Geometry: final body of the model. Coordinates: model frame, mm. Face numbers are marked on the shaded views. A direction names the side the tool comes from. Give positions to 0.01 mm unless a question says otherwise; leave off trailing zeros. Order: outer loops, then holes, each group sorted by start corner. A loop starts at its lowest first (then second) coordinate and runs counter-clockwise, first axis right, second up. Notation, with made-up numbers: (-31, 11) - (21, 11) arc R27 cw to (21, 36) - close; hole circle Ø8 at (51.5, 89.25). An arc over 180 degrees is marked (long way). Put each result on its own line as item: value. Start each with the question number.
1. Ray query, line 1 along Y through (x, z) = (0, -20.25); line 2 along X through (y, z) = (15, 20.5); line 3 along Z through (x, y) = (-3.25, 9.5). Return the intervals inside material, ascending. Write a range as from..to.
2. Set-up query: the marked faces 4 and 5. Return all of +Z, -Z, +X, -X, +Y, -Y with unobstructed straight access to the full face (end or side cutting, diameter ignored); none if empty.
3. First-contact query: P1, Ø2.5, axis at x = 0, y = 8.3, coming from the +Z side; P2, Ø3, axis at x = 3.5, z = -11, coming from the +Y side. Flat tips, straight axial feed; report the tip coordinate or a pass-through.
4. Section B-B on y = 17.5. Return the cut outline in (x, z), plus the area to 3 significant figures.
5. Section C-C on y = 15. Return the cut outline in (x, z), plus the area to 3 significant figures.
6. Section A-A on x = 0. Return the cut outline in (y, z), plus the area to 3 significant figures.
7. Mould query, pull axis Z, two halves, no side actions, for the marked faces 1, 2 and 3. Classes: pulls with the +Z half, pulls with the -Z half, needs draft (parallel to the pull), parting line crosses it, or undercut.
8. Section D-D on x = 3.5. Return the cut outline in (y, z).
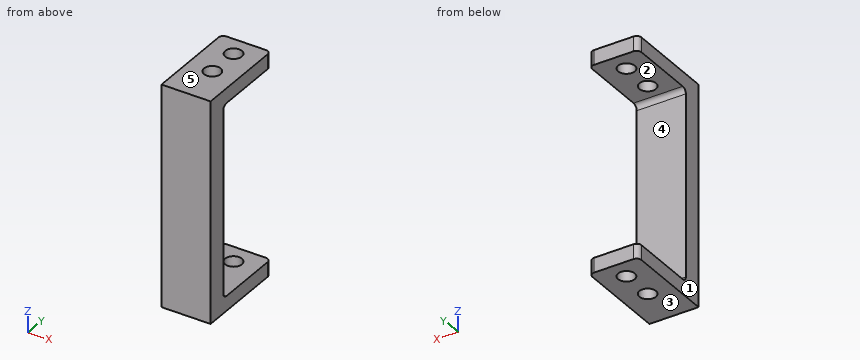
from build123d import *

# Parameters (mm, degrees)
SKETCH2_W                      = 10
SKETCH2_H                      = 45
BOSS_EXTRUDE1_DEPTH            = 4
SKETCH3_W                      = 10
SKETCH3_H                      = 3
BOSS_EXTRUDE2_DEPTH            = 15
M3_CLEARANCE_HOLE1_D           = 3.4
M3_CLEARANCE_HOLE1_ON_FACE_2_D = 3.4
FILLET1_R                      = 1


with BuildPart() as part:
    # Sketch2 → Boss-Extrude1 (new body)
    with BuildSketch(Plane(origin=(0, 0, 0), x_dir=(1, 0, 0), z_dir=(0, 1, 0))):
        Rectangle(SKETCH2_W, SKETCH2_H)
    extrude(amount=BOSS_EXTRUDE1_DEPTH)

    # Sketch3 → Boss-Extrude2 (add)
    with BuildSketch(Plane(origin=(0, 4, 0), x_dir=(1, 0, 0), z_dir=(0, 1, 0))):
        with Locations((0, 21)):
            Rectangle(SKETCH3_W, SKETCH3_H)
        with Locations((0, -21)):
            Rectangle(SKETCH3_W, SKETCH3_H)
    extrude(amount=BOSS_EXTRUDE2_DEPTH)

    # M3 Clearance Hole1 (through all)
    with Locations(Plane(origin=(0, 15, -22.5), x_dir=(-1, 0, 0), z_dir=(0, 0, -1))):
        with Locations((0, 0), (0, -6.7)):
            Hole(M3_CLEARANCE_HOLE1_D / 2)

    # M3 Clearance Hole1 on face 2 (through all)
    with Locations(Plane(origin=(0, 15, 22.5), x_dir=(1, 0, 0), z_dir=(0, 0, 1))):
        with Locations((0, 0), (0, -6.7)):
            Hole(M3_CLEARANCE_HOLE1_ON_FACE_2_D / 2)

    # Fillet1
    fillet1_edges = [part.edges().sort_by_distance(p)[0] for p in [
        (0, 4, -19.5),
        (-5, 19, -21),
        (5, 19, -21),
        (0, 4, 19.5),
        (5, 19, 21),
        (-5, 19, 21),
    ]]
    fillet(fillet1_edges, radius=FILLET1_R)


solid = part.part
Resolved:
1. line 1: 0..6.6, 10..13.3, 16.7..19
1. line 2: -5..-1.7, 1.7..5
1. line 3: -22.5..-19.5, 19.5..22.5
2. face 4: +X, -X, +Y
2. face 5: +Z, +X, -X, +Y, -Y
3. P1: through
3. P2: y = 4
4. outline: (-5, -22.5) - (5, -22.5) - (5, -19.5) - (-5, -19.5) - close; (-5, 19.5) - (5, 19.5) - (5, 22.5) - (-5, 22.5) - close
4. area: 60.0 mm^2
5. outline: (-5, -22.5) - (-1.7, -22.5) - (-1.7, -19.5) - (-5, -19.5) - close; (-5, 19.5) - (-1.7, 19.5) - (-1.7, 22.5) - (-5, 22.5) - close; (1.7, -22.5) - (5, -22.5) - (5, -19.5) - (1.7, -19.5) - close; (1.7, 19.5) - (5, 19.5) - (5, 22.5) - (1.7, 22.5) - close
5. area: 39.6 mm^2
6. outline: (0, -22.5) - (6.6, -22.5) - (6.6, -19.5) - (5, -19.5) arc R1 cw to (4, -18.5) - (4, 18.5) arc R1 cw to (5, 19.5) - (6.6, 19.5) - (6.6, 22.5) - (0, 22.5) - close; (10, -22.5) - (13.3, -22.5) - (13.3, -19.5) - (10, -19.5) - close; (10, 19.5) - (13.3, 19.5) - (13.3, 22.5) - (10, 22.5) - close; (16.7, -22.5) - (19, -22.5) - (19, -19.5) - (16.7, -19.5) - close; (16.7, 19.5) - (19, 19.5) - (19, 22.5) - (16.7, 22.5) - close
6. area: 230 mm^2
7. face 1: needs draft
7. face 2: undercut
7. face 3: pulls with the -Z half
8. outline: (0, -22.5) - (19, -22.5) - (19, -19.5) - (5, -19.5) arc R1 cw to (4, -18.5) - (4, 18.5) arc R1 cw to (5, 19.5) - (19, 19.5) - (19, 22.5) - (0, 22.5) - close
